Geometry check sheet. Reference: the model listing, model coordinates, mm. A direction names the side the tool comes from. Round coordinates to 2 decimals unless told otherwise and drop trailing zeros. Write each loop counter-clockwise with the first axis right and the second up, starting at its lowest first coordinate (ties: lowest second). Pieces come first, ordered by that corner, then holes.
Item 1: Scan lines: probe 1 along X at (y, z) = (1.5, 0); probe 2 along Y at (x, z) = (-2.75, -4); probe 3 along X at (y, z) = (12, -3.5). Record each from-to range of solid material in increasing order.
Item 2: Cross-section at D-D (z = 3.75). Enter the section's corners in (x, y).
Item 3: Depth check by flat-ended pin: P1, Ø1, axis at x = -5.5, z = -4, coming from the +Y side; P2, Ø1.5, axis at y = 11.5, z = -4, coming from the -X side. Enter the tip coordinate at first touch or a pass-through.
Item 4: Cross-section at C-C (z = 0). Enter the section's corners in (x, y), then the cut area to 3 significant figures.
Item 5: Cross-section at A-A (x = -8). Enter the section's corners in (y, z), then the cut area to 3 significant figures.
Item 6: Draft check along Y on faces 3 (the face through (11.41, 18.47, -0.65)), 4 (the face through (11, 25.4, 0)), 5 (the face through (12.7, 13, 0)), 6 (the face through (0, 0, 0)). Enter one of: pulls with the +Y half, pulls with the -Y half, needs draft (parallel to the pull), parting line crosses it, or undercut.
Item 7: Access from +Z, -Z, +X, -X, +Y, -Y to the whole of each face (thin tool, end or side, straight path). Record for faces 1 (the face through (10.16, 14, 0)), 2 (the face through (5, 2, 6.35)).
Item 8: Cross-section at B-B (y = 21.4). Enter the section's corners in (x, z), then the cut area to 3 significant figures.
from build123d import *

# Parameters (mm, degrees)
SKETCH1_W           = 25.4
SKETCH1_H           = 12.7
BOSS_EXTRUDE1_DEPTH = 2.54
SKETCH2_W           = 2.54
SKETCH2_H           = 12.7
BOSS_EXTRUDE2_DEPTH = 22.86
SKETCH3_R           = 3
CUT_EXTRUDE1_DEPTH  = 22.86
SKETCH4_R           = 3
CUT_EXTRUDE2_DEPTH  = 22.86


with BuildPart() as part:
    # Sketch1 → Boss-Extrude1 (new body)
    with BuildSketch(Plane(origin=(0, 0, 0), x_dir=(1, 0, 0), z_dir=(0, 1, 0))):
        Rectangle(SKETCH1_W, SKETCH1_H)
    extrude(amount=BOSS_EXTRUDE1_DEPTH)

    # Sketch2 → Boss-Extrude2 (add)
    with BuildSketch(Plane(origin=(0, 2.54, 0), x_dir=(1, 0, 0), z_dir=(0, 1, 0))):
        with Locations((11.43, 0)):
            Rectangle(SKETCH2_W, SKETCH2_H)
    extrude(amount=BOSS_EXTRUDE2_DEPTH)

    # Sketch3 → Cut-Extrude1 (cut)
    with BuildSketch(Plane(origin=(0, 2.54, 0), x_dir=(1, 0, 0), z_dir=(0, 1, 0))):
        with Locations((-8, 0)):
            Circle(SKETCH3_R)
    extrude(amount=-CUT_EXTRUDE1_DEPTH, mode=Mode.SUBTRACT)

    # Sketch4 → Cut-Extrude2 (cut)
    with BuildSketch(Plane.ZY.offset(-10.16)):
        with Locations((0, 21.4)):
            Circle(SKETCH4_R)
    extrude(amount=-CUT_EXTRUDE2_DEPTH, mode=Mode.SUBTRACT)


solid = part.part
Resolved:
1. probe 1: x = -12.7 to -11, -5 to 12.7
1. probe 2: y = 0 to 2.54
1. probe 3: x = 10.16 to 12.7
2. outline: (-12.7, 0) - (12.7, 0) - (12.7, 25.4) - (10.16, 25.4) - (10.16, 2.54) - (-12.7, 2.54) - close
3. P1: stops at y = 2.54
3. P2: stops at x = 10.16
4. outline: (-12.7, 0) - (-11, 0) - (-11, 2.54) - (-12.7, 2.54) - close; (-5, 0) - (12.7, 0) - (12.7, 18.4) - (10.16, 18.4) - (10.16, 2.54) - (-5, 2.54) - close; (10.16, 24.4) - (12.7, 24.4) - (12.7, 25.4) - (10.16, 25.4) - close
4. area: 92.1 mm2
5. outline: (0, -6.35) - (2.54, -6.35) - (2.54, -3) - (0, -3) - close; (0, 3) - (2.54, 3) - (2.54, 6.35) - (0, 6.35) - close
5. area: 17.0 mm2
6. face 3: undercut
6. face 4: pulls with the +Y half
6. face 5: needs draft
6. face 6: pulls with the -Y half
7. face 1: +Z, -Z, -X, +Y
7. face 2: +Z, +X, -X, +Y, -Y
8. outline: (10.16, -6.35) - (12.7, -6.35) - (12.7, -3) - (10.16, -3) - close; (10.16, 3) - (12.7, 3) - (12.7, 6.35) - (10.16, 6.35) - close
8. area: 17.0 mm2
